Design review of the part built by this model. Coordinates are the model's own, in mm. A direction names the side the tool comes from. Coordinates: 2 decimals unless noted, no trailing zeros. Loops run counter-clockwise (first coordinate to the right, second up) from the corner with the lowest first, then second, coordinate; pieces in that order, holes last.
from build123d import *

# Parameters (mm, degrees)
BASE_FLANGE1_START                    = -1
BASE_FLANGE1_DEPTH                    = 22
SKETCH37_W                            = 8
SKETCH37_H                            = 30
BOSS_EXTRUDE1_DEPTH                   = 1.25
TAP_DRILL_FOR_M4X0_7_TAP1_D           = 3.3
TAP_DRILL_FOR_M4X0_7_TAP1_DEPTH       = 10
TAP_DRILL_FOR_M4X0_7_TAP1_CSINK_D     = 3.35
TAP_DRILL_FOR_M4X0_7_TAP1_CSINK_ANGLE = 90
TAP_DRILL_FOR_M4X0_7_TAP1_TIP         = 0.991420021
SKETCH36_R                            = 1.5
CUT_EXTRUDE1_DEPTH                    = 10


# Read off the part's stored shape, not the designer's step: Base-Flange1
with BuildPart() as part:
    # Base-Flange1 outline → Base-Flange1 (new body)
    with BuildSketch(Plane.XY.offset(BASE_FLANGE1_START)):
        with BuildLine():
            Line((-45.506078027, 0), (-37.492678027, 0))
            Line((-37.492678027, 0), (-37.492678027, 1.25))
            Line((-37.492678027, 1.25), (-45.506078027, 1.25))
            ThreePointArc((-45.506078027, 1.25), (-46.026932882, 1.465745145), (-46.242678027, 1.9866))
            Line((-46.242678027, 1.9866), (-46.242678027, 27.195908555))
            ThreePointArc((-46.242678027, 27.195908555), (-46.216121498, 27.391913221), (-46.138366789, 27.573784833))
            ThreePointArc((-46.138366789, 27.573784833), (0, 53.75), (46.138366789, 27.573784833))
            ThreePointArc((46.138366789, 27.573784833), (46.216121498, 27.391913221), (46.242678027, 27.195908555))
            Line((46.242678027, 27.195908555), (46.242678027, 1.9866))
            ThreePointArc((46.242678027, 1.9866), (46.026932882, 1.465745145), (45.506078027, 1.25))
            Line((45.506078027, 1.25), (37.492678027, 1.25))
            Line((37.492678027, 1.25), (37.492678027, 0))
            Line((37.492678027, 0), (45.506078027, 0))
            ThreePointArc((45.506078027, 0), (46.910816359, 0.581861668), (47.492678027, 1.9866))
            Line((47.492678027, 1.9866), (47.492678027, 27.195908555))
            ThreePointArc((47.492678027, 27.195908555), (47.421055437, 27.724530423), (47.211352064, 28.215035643))
            ThreePointArc((47.211352064, 28.215035643), (0, 55), (-47.211352064, 28.215035643))
            ThreePointArc((-47.211352064, 28.215035643), (-47.421055437, 27.724530423), (-47.492678027, 27.195908555))
            Line((-47.492678027, 27.195908555), (-47.492678027, 1.9866))
            ThreePointArc((-47.492678027, 1.9866), (-46.910816359, 0.581861668), (-45.506078027, 0))
        make_face()
    extrude(amount=BASE_FLANGE1_DEPTH)

    # Sketch37 → Boss-Extrude1 (add)
    with BuildSketch(Plane(origin=(0, 1.25, 0), x_dir=(1, 0, 0), z_dir=(0, 1, 0))):
        with Locations((41.492678027, -36)):
            Rectangle(SKETCH37_W, SKETCH37_H)
        with Locations((-41.492678027, -36)):
            Rectangle(SKETCH37_W, SKETCH37_H)
    extrude(amount=-BOSS_EXTRUDE1_DEPTH)

    # Tap Drill for M4x0.7 Tap1
    with Locations(Plane(origin=(0, 1.25, 0), x_dir=(1, 0, 0), z_dir=(0, 1, 0))):
        with Locations((-42.455982414, -35.991709022), (42.455982414, -35.991709022)):
            CounterSinkHole(TAP_DRILL_FOR_M4X0_7_TAP1_D / 2, TAP_DRILL_FOR_M4X0_7_TAP1_CSINK_D / 2, depth=TAP_DRILL_FOR_M4X0_7_TAP1_DEPTH, counter_sink_angle=TAP_DRILL_FOR_M4X0_7_TAP1_CSINK_ANGLE)
            with Locations((0, 0, -(TAP_DRILL_FOR_M4X0_7_TAP1_DEPTH + TAP_DRILL_FOR_M4X0_7_TAP1_TIP / 2))):  # 118° drill point
                Cone(0, TAP_DRILL_FOR_M4X0_7_TAP1_D / 2, TAP_DRILL_FOR_M4X0_7_TAP1_TIP, mode=Mode.SUBTRACT)

    # Sketch36 → Cut-Extrude1 (cut)
    with BuildSketch(Plane(origin=(0, 1.25, 0), x_dir=(1, 0, 0), z_dir=(0, 1, 0))):
        with Locations(Location((42.000000004, -2, 0), (0, 0, 180))):
            Circle(SKETCH36_R)
        with Locations(Location((-42.000000004, -2, 0), (0, 0, 270))):
            Circle(SKETCH36_R)
    extrude(amount=-CUT_EXTRUDE1_DEPTH, mode=Mode.SUBTRACT)


solid = part.part
Q1. Take a section at D-D, the plane x = 22. Write out the cut boundary in (y, z), then the cut area to 3 significant figures.
Q2. Take a section at C-C, the plane z = 43.5. Write out the cut boundary in (x, y), then the cut area to 3 significant figures.
Q3. Machinability: for faces 1 (the cylindrical face through (-43.464, 0.634, 1.675)), 2 (the cylindrical face through (0.795, 54.994, 9.846)), 3 (the flat face through (-46.243, 14, 10)), which of the approach directions +Z, -Z, +X, -X, +Y, -Y give a long, thin tool a straight path to every point of the face, cutting with its end or side? Answer none if there is none.
Q4. Clearance check with flat-ended pins moving along their axes: pin 1 Ø9 at (x, z) = (-41.5, 23) entering from +Y; pin 2 Ø5.5 at (x, z) = (-42.46, 35.99) entering from +Y; pin 3 Ø0.6 at (y, z) = (0.5, 27) entering from +X; pin 4 Ø2 at (x, z) = (42.46, 35.99) entering from -Y. State where each tip first meets the part, or that it passes through.
Q5. For line 1 (X direction, y = 3, z = 18); line 2 (Y direction, x = 41, z = 41.5); line 3 (X direction, y = 49, z = 7.5), list the stretches that pass through material, from the lowest coordinate up.
Q6. Take a section at B-B, the plane z = 2. Write out the cut boundary in (x, y).
Q7. Take a section at A-A, the plane y = 10.5. Write out the cut boundary in (x, z), then the cut area to 3 significant figures.
Q8. The part is to be moulded in two halves that separate along X. For faces 4 (the flat face through (41, 0, 25)), 5 (the cylindrical face through (-0.777, 53.744, 9.846)), 6 (the flat face through (46.243, 15, 10)), 7 (the cylindrical face through (46.9, 0.57, 9.85)), say which applies: pulls with the +X half, pulls with the -X half, needs draft (parallel to the pull), parting line crosses it, or undercut.
Entries:
1. outline: (49.04, -1) - (50.41, -1) - (50.41, 21) - (49.04, 21) - close
1. area: 30.1 mm2
2. outline: (-45.49, 0) - (-37.49, 0) - (-37.49, 1.25) - (-45.49, 1.25) - close; (37.49, 0) - (45.49, 0) - (45.49, 1.25) - (37.49, 1.25) - close
2. area: 20.0 mm2
3. face 1: -Y
3. face 2: +Z, -Z, +Y
3. face 3: +Z, -Z
4. pin 1: stops at y = 40.26
4. pin 2: stops at y = 1.25
4. pin 3: stops at x = 45.49
4. pin 4: passes through
5. line 1: x = -47.49 to -46.24, 46.24 to 47.49
5. line 2: y = 0 to 1.25
5. line 3: x = -24.98 to -22.09, 22.09 to 24.98
6. outline: (-47.49, 1.99) arc R1.99 ccw to (-45.51, 0) - (-43.5, 0) - (-43.5, 1.25) - (-45.51, 1.25) arc R0.74 cw to (-46.24, 1.99) - (-46.24, 27.2) arc R0.74 cw to (-46.14, 27.57) arc R53.75 cw to (46.14, 27.57) arc R0.74 cw to (46.24, 27.2) - (46.24, 1.99) arc R0.74 cw to (45.51, 1.25) - (43.5, 1.25) - (43.5, 0) - (45.51, 0) arc R1.99 ccw to (47.49, 1.99) - (47.49, 27.2) arc R1.99 ccw to (47.21, 28.22) arc R55 ccw to (-47.21, 28.22) arc R1.99 ccw to (-47.49, 27.2) - close; (-40.5, 0) - (-37.49, 0) - (-37.49, 1.25) - (-40.5, 1.25) - close; (37.49, 0) - (40.5, 0) - (40.5, 1.25) - (37.49, 1.25) - close
7. outline: (-47.49, -1) - (-46.24, -1) - (-46.24, 21) - (-47.49, 21) - close; (46.24, -1) - (47.49, -1) - (47.49, 21) - (46.24, 21) - close
7. area: 55.0 mm2
8. face 4: needs draft
8. face 5: undercut
8. face 6: undercut
8. face 7: pulls with the +X half
